Verification items for the finished model (mm, model axes). Face numbers are marked on the shaded views. Give positions to 0.01 mm unless a question says otherwise; leave off trailing zeros. Write each loop counter-clockwise with the first axis right and the second up, starting at its lowest first coordinate (ties: lowest second). Pieces come first, ordered by that corner, then holes. Notation, with made-up numbers: (9, -37.5) - (36, -37.5) arc R23 cw to (36, -4.5) - close; hole circle Ø10 at (4, 70). An arc over 180 degrees is marked (long way). Put each result on its own line as item: value.
Autodesk Inventor part; units mm, degrees
sketch "Sketch1" plane through (0, 0, 0) normal (0, 0, 1) x (1, 0, 0)
  line L0 (-23.5, 7.5) -> (23.5, 7.5)
  line L1 (23.5, 7.5) -> (23.5, -7.5)
  line L2 (23.5, -7.5) -> (-23.5, -7.5)
  line L3 (-23.5, -7.5) -> (-23.5, 7.5)
  line L4 (-23.5, 7.5) -> (23.5, -7.5) construction
  line L5 (23.5, 7.5) -> (-23.5, -7.5) construction
  circle A0 centre (17, 0) radius 2.5
  circle A1 centre (8, 2.5) radius 1
  circle A2 centre (8, -2.5) radius 1
  line L6 (8, 2.5) -> (8, -2.5) construction
  line L7 (0, 7.5) -> (0, -7.5) construction
  circle A3 centre (-17, 0) radius 2.5
  circle A4 centre (-8, 2.5) radius 1
  circle A5 centre (-8, -2.5) radius 1
  point P0 (0, 0)
  point P1 (0, 0)
  point P2 (8, 0)
  point P3 (0, 0)
  dimension "d0" = 47
  dimension "d1" = 15
  dimension "d6" = 5
  dimension "d7" = 17
  dimension "d8" = 2
  dimension "d9" = 2
  dimension "d10" = 8
  dimension "d11" = 5
extrude "Extrusion1" add sketch "Sketch1" along normal mid plane 10
properties part number "suporte_motor_001" material "ABS Plastic"
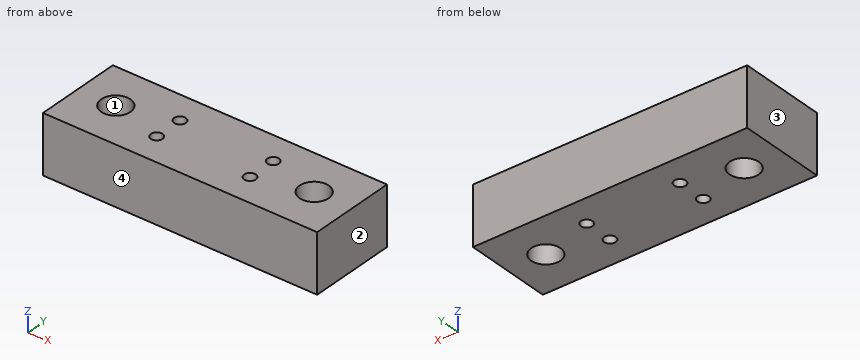
Q1. Section check B-B, the plane x = 17. Record the cut outline in (y, z).
Answers follow:
outline: (-7.5, -5) - (-2.5, -5) - (-2.5, 5) - (-7.5, 5) - close; (2.5, -5) - (7.5, -5) - (7.5, 5) - (2.5, 5) - close
Q2. Release check for a two-part mould opening along X. For the marked faces 1, 2, 3 and 4 record: released by +X, released by -X, zero draft, split by the parting line, or undercut.
Answers follow:
face 1: undercut
face 2: released by +X
face 3: released by -X
face 4: zero draft
Q3. Section check A-A, the plane y = 0. Record the cut outline in (x, z).
Answers follow:
outline: (-23.5, -5) - (-19.5, -5) - (-19.5, 5) - (-23.5, 5) - close; (-14.5, -5) - (14.5, -5) - (14.5, 5) - (-14.5, 5) - close; (19.5, -5) - (23.5, -5) - (23.5, 5) - (19.5, 5) - close
Q4. Scan lines: line 1 along Y through (x, z) = (8, -2); line 2 along Y through (x, z) = (7.5, 1.75); line 3 along Y through (x, z) = (-17, -2). Record each from-to range of solid material in increasing order.
Answers follow:
line 1: y = -7.5 to -3.5, -1.5 to 1.5, 3.5 to 7.5
line 2: y = -7.5 to -3.37, -1.63 to 1.63, 3.37 to 7.5
line 3: y = -7.5 to -2.5, 2.5 to 7.5
Q5. Section check D-D, the plane x = 8. Record the cut outline in (y, z).
Answers follow:
outline: (-7.5, -5) - (-3.5, -5) - (-3.5, 5) - (-7.5, 5) - close; (-1.5, -5) - (1.5, -5) - (1.5, 5) - (-1.5, 5) - close; (3.5, -5) - (7.5, -5) - (7.5, 5) - (3.5, 5) - close
Q6. Section check C-C, the plane z = -3.25. Record the cut outline in (x, y), plus the area to 3 significant figures.
Answers follow:
outline: (-23.5, -7.5) - (23.5, -7.5) - (23.5, 7.5) - (-23.5, 7.5) - close; hole circle Ø5 at (-17, 0); hole circle Ø2 at (-8, -2.5); hole circle Ø2 at (-8, 2.5); hole circle Ø2 at (8, -2.5); hole circle Ø2 at (8, 2.5); hole circle Ø5 at (17, 0)
area: 653 mm2
Q7. Go/stop test with a flat-tipped pin: pin 1 Ø4.5 at (x, y) = (-17, 0) entering from -Z. Record where the tip stops, or that it passes through.
Answers follow:
pin 1: passes through
